Model file for the job. Use its own axes, mm. A direction names the side the tool comes from. Give positions to 0.01 mm unless a question says otherwise; leave off trailing zeros. Write each loop counter-clockwise with the first axis right and the second up, starting at its lowest first coordinate (ties: lowest second). Pieces come first, ordered by that corner, then holes.
```python
from build123d import *

# Parameters (mm, degrees)
F0_W     = 101.6
F0_H     = 101.6
F0_R     = 9.525
F1_DEPTH = 6.35
F2_W     = 6.35
F2_H     = 30.48
F3_DEPTH = 25.4
F4_W     = 6.35
F4_H     = 15.24
F7_R     = 3.175
F8_DEPTH = 44.45


with BuildPart() as f1:
    # F0 (on Top) → F1 (new body)
    with BuildSketch(Plane.XY):
        Rectangle(F0_W, F0_H)
        with Locations((-28.575, -28.575)):
            Circle(F0_R, mode=Mode.SUBTRACT)
        with Locations((28.575, -28.575)):
            Circle(F0_R, mode=Mode.SUBTRACT)
        with Locations((-28.575, 28.575)):
            Circle(F0_R, mode=Mode.SUBTRACT)
        with Locations((28.575, 28.575)):
            Circle(F0_R, mode=Mode.SUBTRACT)
    extrude(amount=F1_DEPTH)

    # F2 (on face) → F3 (join)
    with BuildSketch(Plane.XY.offset(6.35)):
        with Locations((15.875, 0)):
            Rectangle(F2_W, F2_H)
        with Locations((-15.875, 0)):
            Rectangle(F2_W, F2_H)
    extrude(amount=F3_DEPTH)

    # F4 (on face) → F5 (revolve)
    with BuildSketch(Plane.XY.offset(31.75)):
        with Locations((15.875, -7.62)):
            Rectangle(F4_W, F4_H)
    revolve(axis=Axis((15.875, 0, 31.75), (1, 0, 0)))

    # F6: F1 across plane


with BuildPart() as f1_1:
    add(f1.part)
    add(f1.part.mirror(Plane.YZ))

    # F7 (on face) → F8 (cut)
    with BuildSketch(Plane.YZ.offset(19.05)):
        with Locations((0, 31.75)):
            Circle(F7_R)
    extrude(amount=-F8_DEPTH, mode=Mode.SUBTRACT)


solid = f1_1.part
```
1. Slice it at B-B, the plane y = 0. Write the cut outline in (x, z) (3 decimals).
Calculated:
outline: (-50.8, 0) - (50.8, 0) - (50.8, 6.35) - (19.05, 6.35) - (19.05, 28.575) - (12.7, 28.575) - (12.7, 6.35) - (-12.7, 6.35) - (-12.7, 28.575) - (-19.05, 28.575) - (-19.05, 6.35) - (-50.8, 6.35) - close; (-19.05, 34.925) - (-12.7, 34.925) - (-12.7, 46.99) - (-19.05, 46.99) - close; (12.7, 34.925) - (19.05, 34.925) - (19.05, 46.99) - (12.7, 46.99) - close
2. Slice it at D-D, the plane z = 33. Write the cut outline in (x, y).
Calculated:
outline: (-19.05, -15.19) - (-12.7, -15.19) - (-12.7, -2.92) - (-19.05, -2.92) - close; (-19.05, 2.92) - (-12.7, 2.92) - (-12.7, 15.19) - (-19.05, 15.19) - close; (12.7, -15.19) - (19.05, -15.19) - (19.05, -2.92) - (12.7, -2.92) - close; (12.7, 2.92) - (19.05, 2.92) - (19.05, 15.19) - (12.7, 15.19) - close
3. Probe probe 1 along Z at (x, y) = (15, 0) (3 decimals); probe 2 along X at (y, z) = (5, 10); probe 3 along X at (y, z) = (32.5, 6). List the from-to ranges inside material, lowest first.
Calculated:
probe 1: z = 0 to 28.575, 34.925 to 46.99
probe 2: x = -19.05 to -12.7, 12.7 to 19.05
probe 3: x = -50.8 to -37.25, -19.9 to 19.9, 37.25 to 50.8
4. Which spindle directions (+Z, -Z, +X, -X, +Y, -Y) get a long thin tool onto all of the face, cutting with end or side? Do faces 4 (the flat face through (12.7, 0, 26)), 5 (the flat face through (16, -15.24, 19)), 6 (the flat face through (16, 15.24, 19)). Say none if no direction does.
Calculated:
face 4: +Z, +Y, -Y
face 5: +Z, +X, -X, -Y
face 6: +Z, +X, -X, +Y
5. Slice it at A-A, the plane z = 22.5. Write the cut outline in (x, y), and give its area (3 significant figures).
Calculated:
outline: (-19.05, -15.24) - (-12.7, -15.24) - (-12.7, 15.24) - (-19.05, 15.24) - close; (12.7, -15.24) - (19.05, -15.24) - (19.05, 15.24) - (12.7, 15.24) - close
area: 387 mm2
6. Pull direction X, two halves, no side cores. Call faces 1 (the flat face through (-12.7, 0, 26)), 2 (the flat face through (-50.8, -1, 3)), 3 (the flat face through (-1, 1, 0)): +X half, -X half, draft (parallel to the pull), parting line (faces both ways), or undercut.
Calculated:
face 1: undercut
face 2: -X half
face 3: draft
7. Pin check, flat tips, straight feed: P1, Ø10, axis at y = 0, z = 31.75, coming from the -X side; P2, Ø15, axis at y = -0.5, z = 28.5, coming from the +X side; P3, Ø1.9, axis at x = -16, z = 17.5, coming from the +Y side; P4, Ø10, axis at x = 22.5, y = 19.5, coming from the -Z side. Stop position of each tip, or through.
Calculated:
P1: stops at x = -19.05
P2: stops at x = 19.05
P3: stops at y = 15.24
P4: stops at z = 0
8. Slice it at C-C, the plane x = -26. Write the cut outline in (y, z), and give its area (3 significant figures).
Calculated:
outline: (-50.8, 0) - (-37.75, 0) - (-37.75, 6.35) - (-50.8, 6.35) - close; (-19.4, 0) - (19.4, 0) - (19.4, 6.35) - (-19.4, 6.35) - close; (37.75, 0) - (50.8, 0) - (50.8, 6.35) - (37.75, 6.35) - close
area: 412 mm2
